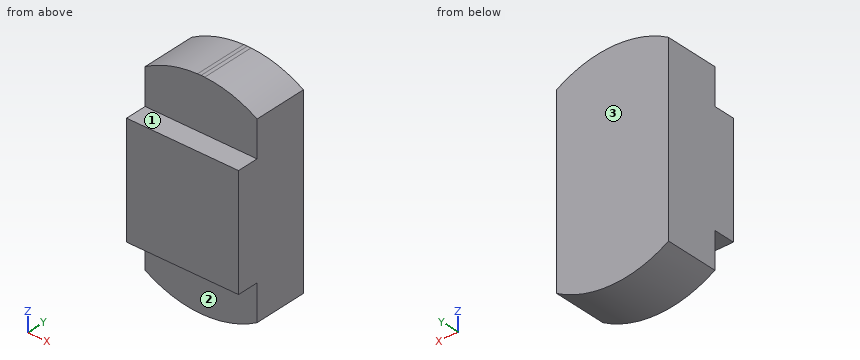
```python
from build123d import *

# Parameters (mm, degrees)
F0_R      = 12.7
F1_DEPTH  = 10
F1_FACE_W = 52
F1_FACE_H = 52
F2_DEPTH  = 25


with BuildPart() as f1:
    # F0 (on Front) → F1 (new body)
    with BuildSketch(Plane.XZ):
        with BuildLine():
            Line((-26, -26), (0, -26))
            ThreePointArc((0, -26), (-18.384776, -18.384776), (-26, 0))
            Line((-26, 0), (-26, -26))
        make_face()
        with BuildLine():
            Line((26, -26), (26, 0))
            ThreePointArc((26, 0), (18.384776, -18.384776), (0, -26))
            Line((0, -26), (26, -26))
        make_face()
        with BuildLine():
            ThreePointArc((-26, 0), (-18.384776, 18.384776), (0, 26))
            Line((0, 26), (-26, 26))
            Line((-26, 26), (-26, 0))
        make_face()
        with BuildLine():
            ThreePointArc((0, 26), (18.384776, 18.384776), (26, 0))
            Line((26, 0), (26, 26))
            Line((26, 26), (0, 26))
        make_face()
        with BuildLine():
            ThreePointArc((0, -26), (18.384776, -18.384776), (26, 0))
            ThreePointArc((26, 0), (18.384776, 18.384776), (0, 26))
            ThreePointArc((0, 26), (-18.384776, 18.384776), (-26, 0))
            ThreePointArc((-26, 0), (-18.384776, -18.384776), (0, -26))
        make_face()
        Circle(F0_R, mode=Mode.SUBTRACT)
        Circle(F0_R)
    extrude(amount=F1_DEPTH)

    # F0 (on Front) + F1_face (on face) → F2 (join)
    with BuildSketch(Plane.XZ):
        with BuildLine():
            Line((26, -26), (26, 0))
            ThreePointArc((26, 0), (18.384776, -18.384776), (0, -26))
            Line((0, -26), (26, -26))
        make_face()
        with BuildLine():
            ThreePointArc((0, 26), (18.384776, 18.384776), (26, 0))
            Line((26, 0), (26, 26))
            Line((26, 26), (0, 26))
        make_face()
        with BuildLine():
            Line((-26, 26), (0, 26))
            Line((0, 26), (26, 26))
            Line((26, 26), (26, 42.708313))
            ThreePointArc((26, 42.708313), (14.304673, 47.910086), (1.67188, 49.97204))
            Line((1.67188, 49.97204), (0, 50.027975))
            Line((0, 50.027975), (-1.67188, 49.97204))
            ThreePointArc((-1.67188, 49.97204), (-14.304673, 47.910086), (-26, 42.708313))
            Line((-26, 42.708313), (-26, 26))
        make_face()
        with BuildLine():
            ThreePointArc((-26, 0), (-18.384776, 18.384776), (0, 26))
            Line((0, 26), (-26, 26))
            Line((-26, 26), (-26, 0))
        make_face()
        with BuildLine():
            Line((-26, -26), (0, -26))
            ThreePointArc((0, -26), (-18.384776, -18.384776), (-26, 0))
            Line((-26, 0), (-26, -26))
        make_face()
        with BuildLine():
            Line((26, -26), (0, -26))
            Line((0, -26), (-26, -26))
            Line((-26, -26), (-26, -42.708313))
            ThreePointArc((-26, -42.708313), (0, -50), (26, -42.708313))
            Line((26, -42.708313), (26, -26))
        make_face()
    with BuildSketch(Plane.XZ.offset(10)):
        Rectangle(F1_FACE_W, F1_FACE_H)
    extrude(amount=F2_DEPTH)


solid = f1.part
```
For this review, take the finished solid that the model builds, in its own axes (mm). Face numbers are marked on the shaded views. A direction names the side the tool comes from. Give positions to 0.01 mm unless a question says otherwise; leave off trailing zeros. Write each loop counter-clockwise with the first axis right and the second up, starting at its lowest first coordinate (ties: lowest second). Pieces come first, ordered by that corner, then holes. Notation, with made-up numbers: M 76,13.5 L 92,13.5 A19 cw 92,21.5 Z; hole C 57.25,14 d4. An arc over 180 degrees is marked long. Answer as a JSON object with one key per item and string values. Group by question number.
Item 1: For pin 1 Ø4 at (x, y) = (-5, -6) entering from -Z; pin 2 Ø1.5 at (x, y) = (15, -5.5) entering from -Z; pin 3 Ø10 at (x, y) = (-13.5, -27.5) entering from -Z, all flat-tipped, find the tip position at first contact; note any pin that passes through.
Item 2: Consider section D-D on x = 20. Write out the cut boundary in (y, z).
Item 3: Consider section A-A on y = -3. Write out the cut boundary in (x, z), plus the area to 3 significant figures.
Item 4: For probe 1 along Y at (x, z) = (-18, -27.5); probe 2 along Z at (x, y) = (4, -28.5); probe 3 along Z at (x, y) = (-0.5, -6.5), list the stretches that pass through material, from the lowest coordinate up. Write a range as [from, to].
Item 5: Consider section B-B on x = -12. Write out the cut boundary in (y, z), plus the area to 3 significant figures.
Item 6: Tool access review of the marked faces 1, 2 and 3: name each direction out of +Z, -Z, +X, -X, +Y, -Y from which nothing blocks a thin tool from reaching the whole face with its end or side.
Item 7: Consider section C-C on z = -32. Write out the cut boundary in (x, y), plus the area to 3 significant figures.
Check result:
{
 "1": {"pin 1": "stops at z = -49.91", "pin 2": "stops at z = -47.93", "pin 3": "stops at z = -49.15"},
 "2": {"outline": "M -35,-26 L -25,-26 L -25,-45.83 L 0,-45.83 L 0,45.83 L -25,45.83 L -25,26 L -35,26 Z"},
 "3": {"outline": "M -26,-42.71 A50 ccw 26,-42.71 L 26,42.71 A50 ccw 1.67,49.97 L 0,50.03 L -1.67,49.97 A50 ccw -26,42.71 Z", "area": "4,960 mm^2"},
 "4": {"probe 1": "y = [-25, 0]", "probe 2": "z = [-26, 26]", "probe 3": "z = [-50, 50.01]"},
 "5": {"outline": "M -35,-26 L -25,-26 L -25,-48.54 L 0,-48.54 L 0,48.54 L -25,48.54 L -25,26 L -35,26 Z", "area": "2,950 mm^2"},
 "6": {"face 1": "+Z, +X, -X, -Y", "face 2": "-Z, +X, -X, -Y", "face 3": "+Z, -Z, +X, -X, +Y"},
 "7": {"outline": "M -26,-25 L 26,-25 L 26,0 L -26,0 Z", "area": "1,300 mm^2"}
}
